Geometry check sheet. Reference: the model listing, model coordinates, mm. A direction names the side the tool comes from. Coordinates: 2 decimals unless noted, no trailing zeros. Order: outer loops, then holes, each group sorted by start corner. A loop starts at its lowest first (then second) coordinate and runs counter-clockwise, first axis right, second up. Notation, with made-up numbers: (40.25, 44) - (51.25, 44) arc R31 ccw to (51.25, 81) - close; hole circle Ø2 at (65.5, 50.5). An arc over 180 degrees is marked (long way). Put each result on its own line as item: value.
from build123d import *

# Parameters (mm, degrees)
F1_DEPTH = 25
F3_DEPTH = 200
F6_DEPTH = 25


with BuildPart() as f1:
    # F0 (on Front) → F1 (new body)
    with BuildSketch(Plane.XZ):
        Polygon((0, 200), (0, 100), (450, 100), (575, 316.5063509461), (401.7949192431, 416.5063509461), (276.7949192431, 200), align=None)
    extrude(amount=F1_DEPTH)

    # F2 (on face) → F3 (join)
    with BuildSketch(Plane.XZ.offset(25)):
        with BuildLine():
            ThreePointArc((345.7026108616, 254.0491654437), (357.30455878, 255.6108989307), (362.7, 266))
            ThreePointArc((362.7, 266), (342.69544122, 276.3891010693), (345.7026108616, 254.0491654437))
        make_face()
        with BuildLine():
            ThreePointArc((310.2, 120), (307.8891010693, 127.30455878), (301.7973891384, 131.9508345563))
            ThreePointArc((301.7973891384, 131.9508345563), (287.1108989307, 112.69544122), (310.2, 120))
        make_face()
    extrude(amount=F3_DEPTH)

    # F4: F1 across plane


with BuildPart() as f1_1:
    add(f1.part)
    add(f1.part.mirror(Plane.YZ))

    # F5 (on face) → F6 (join)
    with BuildSketch(Plane.XZ.offset(25)):
        with BuildLine():
            Line((-34.6410161514, 100), (-12.5, 61.6506350946))
            ThreePointArc((-12.5, 61.6506350946), (0, 15), (12.5, 61.6506350946))
            Line((12.5, 61.6506350946), (34.6410161514, 100))
            Line((34.6410161514, 100), (-34.6410161514, 100))
        make_face()
    extrude(amount=-F6_DEPTH)

    # F8 (on line) → F9 (revolve)
    with BuildSketch(Plane(origin=(225.2265575507, 0, -80.989001859), x_dir=(0, -1, 0), z_dir=(-0.941010595, 0, 0.3383770975))):
        with BuildLine():
            Line((25, 328.7408023961), (25, 318.7408023961))
            Line((25, 318.7408023961), (85, 318.7408023961))
            ThreePointArc((85, 318.7408023961), (77.588190451, 328.400060659), (66.3397459622, 323.7408023961))
            Line((66.3397459622, 323.7408023961), (60, 323.7408023961))
            Line((60, 323.7408023961), (60, 328.7408023961))
            Line((60, 328.7408023961), (25, 328.7408023961))
        make_face()
    revolve(axis=Axis((333.0811451244, -55, 218.9494702506), (0, -1, 0)))


solid = f1_1.part
Q1. Section check A-A on y = -171. Record the boundary of the cut face in (x, z).
Answer block:
outline: circle Ø25.4 at (-350, 266); circle Ø25.4 at (-297.5, 120); circle Ø25.4 at (297.5, 120); circle Ø25.4 at (350, 266)
Q2. Section check B-B on z = 360.5. Record the boundary of the cut face in (x, y), then the cut area to 3 significant figures.
Answer block:
outline: (-498.8, -25) - (-369.46, -25) - (-369.46, 0) - (-498.8, 0) - close; (369.46, -25) - (498.8, -25) - (498.8, 0) - (369.46, 0) - close
area: 6,470 mm^2
Q3. Depth check by flat-ended pin: pin 1 Ø10 at (x, y) = (-363, -166) entering from +Z; pin 2 Ø7.5 at (x, y) = (220, -7) entering from -Z; pin 3 Ø1.5 at (x, z) = (-50.5, 197) entering from -Y; pin 4 Ø10 at (x, z) = (353.5, 351.5) entering from +Y. Enter the tip coordinate at first touch or a pass-through.
Answer block:
pin 1: stops at z = 275.86
pin 2: stops at z = 100
pin 3: stops at y = -25
pin 4: passes through
Q4. Draft check along Y on faces 1 (the cylindrical face through (-0.916, -12.675, 15.017)), 2 (the flat face through (-350, -225, 266)), 3 (the flat face through (337, -60, 223)). Enter one of: pulls with the +Y half, pulls with the -Y half, needs draft (parallel to the pull), parting line crosses it, or undercut.
Answer block:
face 1: needs draft
face 2: pulls with the -Y half
face 3: undercut
Q5. Access from +Z, -Z, +X, -X, +Y, -Y to the whole of each face (thin tool, end or side, straight path). Record for faces 4 (the flat face through (-23.725, -12.675, 81.094)), 5 (the cylindrical face through (339.811, -42.255, 226.346)), 6 (the flat face through (245, -12, 100)), 7 (the flat face through (-4, -12, 200)), 8 (the flat face through (23.416, -12.675, 80.557)).
Answer block:
face 4: -X, +Y, -Y
face 5: -Y
face 6: -Z, +X, +Y, -Y
face 7: +Z, +Y, -Y
face 8: +X, +Y, -Y
Q6. Section check D-D on x = -188. Record the boundary of the cut face in (y, z), then the cut area to 3 significant figures.
Answer block:
outline: (-25, 100) - (0, 100) - (0, 200) - (-25, 200) - close
area: 2,500 mm^2
Q7. Section check C-C on y = -37.5. Record the boundary of the cut face in (x, z), then the cut area to 3 significant figures.
Answer block:
outline: circle Ø25.4 at (-350, 266); circle Ø25.4 at (-297.5, 120); circle Ø25.4 at (297.5, 120); circle Ø20 at (333.08, 218.95); circle Ø25.4 at (350, 266)
area: 2,340 mm^2
Q8. Thickness scan on L1, parallel to Y at x = 13, z = 183; L2, parallel to X at y = -112, z = 272; L3, parallel to X at y = -21, z = 309.5. Record the ranges inside material, lowest first. Write a range as [from, to].
Answer block:
L1: y = [-25, 0]
L2: x = [-361.19, -338.81], [338.81, 361.19]
L3: x = [-570.95, -340.01], [340.01, 570.95]
